Geometry check sheet. Reference: drawing and pictorial views, mm from the part's lowest x, y, z. A direction names the side the tool comes from. Round coordinates to 2 decimals unless told otherwise and drop trailing zeros. Write each loop counter-clockwise with the first axis right and the second up, starting at its lowest first coordinate (ties: lowest second). Pieces come first, ordered by that corner, then holes. Notation, with made-up numbers: (12, 9) - (18, 9) arc R6 cw to (18, 16) - close; hole circle Ø1 at (64, 20.5). An arc over 180 degrees is marked (long way). Use one line per item in the form item = value. Start each with the question number.
1) Section check D-D (x = 6.35). Record the boundary of the cut face in (y, z).
2) Section check C-C (z = 17). Record the boundary of the cut face in (x, y).
3) Set-up check for the marked faces 1 and 2: record each of +Z, -Z, +X, -X, +Y, -Y from which the full face is reachable in a straight line by a thin tool's end or side.
4) Scan lines: probe 1 along Z at (x, y) = (31.75, 0.8); probe 2 along Z at (x, y) = (5, 22); probe 3 along Y at (x, z) = (27.5, 1). Record each from-to range of solid material in increasing order.
5) Gauge pin test, flat ends, axial feed: P1, Ø5, axis at x = 12.5, y = 54.5, coming from the +Z side; P2, Ø3.5, axis at x = 13.08, y = 7.51, coming from the +Z side; P3, Ø5, axis at x = 27.5, y = 47.5, coming from the -Z side; P4, Ø10, axis at x = 15.5, z = 15.5, coming from the +Y side. Record the tip position at first contact, or that the pin passes through.
6) Section check B-B (y = 18.5). Record the boundary of the cut face in (x, z).
7) Section check A-A (x = 20). Record the boundary of the cut face in (y, z).
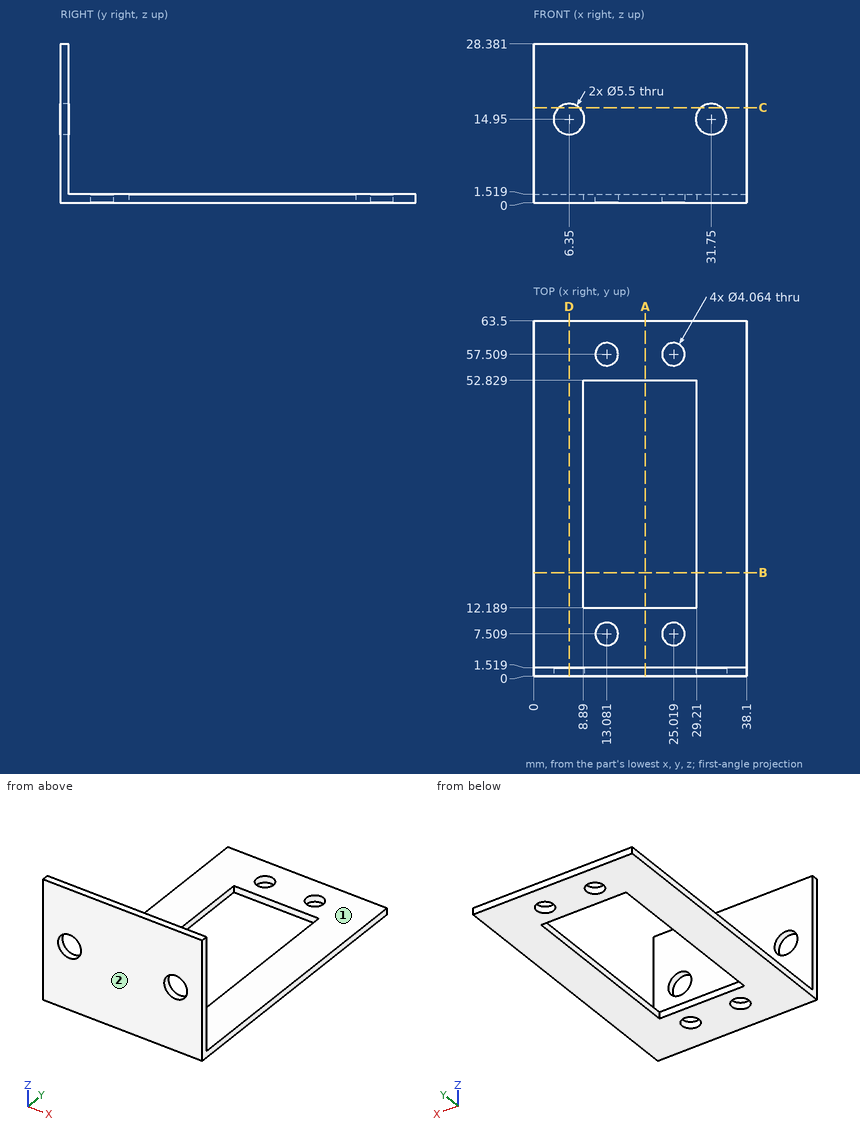
Results are:
q1.outline = (0, 0) - (63.5, 0) - (63.5, 1.52) - (1.52, 1.52) - (1.52, 12.2) - (0, 12.2) - close; (0, 17.7) - (1.52, 17.7) - (1.52, 28.38) - (0, 28.38) - close
q2.outline = (0, 0) - (4.52, 0) - (4.52, 1.52) - (0, 1.52) - close; (8.18, 0) - (29.92, 0) - (29.92, 1.52) - (8.18, 1.52) - close; (33.58, 0) - (38.1, 0) - (38.1, 1.52) - (33.58, 1.52) - close
q3.face_1 = +Z, +X, -X, +Y
q3.face_2 = +Z, -Z, +X, -X, -Y
q4.probe_1 = 0 to 12.2, 17.7 to 28.38
q4.probe_2 = 0 to 1.52
q4.probe_3 = 0 to 12.19, 52.83 to 63.5
q5.P1 = 1.52
q5.P2 = through
q5.P3 = 0
q5.P4 = 1.52
q6.outline = (0, 0) - (8.89, 0) - (8.89, 1.52) - (0, 1.52) - close; (29.21, 0) - (38.1, 0) - (38.1, 1.52) - (29.21, 1.52) - close
q7.outline = (0, 0) - (12.19, 0) - (12.19, 1.52) - (1.52, 1.52) - (1.52, 28.38) - (0, 28.38) - close; (52.83, 0) - (63.5, 0) - (63.5, 1.52) - (52.83, 1.52) - close
